from build123d import *


with BuildPart() as part:
    # Sketch1 → Revolve1 (revolve)
    with BuildSketch(Plane(origin=(0, 0, 0), x_dir=(0, 0, -1), z_dir=(1, 0, 0))):
        Polygon((-562.5, 225), (-562.5, -225), (0, -225), (0, -185), (0, 225), (0, 252.019037432), (-562.5, 252.019037432), align=None)
        Polygon((-30, -190), (-220, -190), (-220, -215), (-275, -215), (-275, -190), (-537.5, -190), (-537.5, 185), (-537.5, 225), (-30, 225), (-30, 185), align=None, mode=Mode.SUBTRACT)
    revolve(axis=Axis((0, 225, 0), (0, -1, 0)))


solid = part.part
The model under review builds one solid part; all positions refer to its coordinate system, in mm. A direction names the side the tool comes from. Round coordinates to 2 decimals unless told otherwise and drop trailing zeros. Loops run counter-clockwise (first coordinate to the right, second up) from the corner with the lowest first, then second, coordinate; pieces in that order, holes last. Notation, with made-up numbers: M 41,67 L 75,67 A10 cw 75,74 Z; hole C -22.75,59.5 d4. An arc over 180 degrees is marked long. Answer as CSV lines item,"result".
1. Insertion check: pin 1 Ø6 at (y, z) = (115.5, -178) entering from -X; pin 2 Ø10 at (x, y) = (170.5, 83.5) entering from +Z; pin 3 Ø12 at (y, z) = (115.5, -367) entering from -X. Each pin has a flat end and moves straight along its axis. Give the tip position at first contact, or say it passes through.
Outcome:
pin 1,"stops at x = -534.59"
pin 2,"stops at z = 537.6"
pin 3,"stops at x = -431.38"
2. We need section D-D (x = 354). Give the boundary of the cut face in (y, z).
Outcome:
outline,"M -225,-437.14 L 252.02,-437.14 L 252.02,437.14 L -225,437.14 Z; hole M -190,-404.46 L 225,-404.46 L 225,404.46 L -190,404.46 Z"
3. We need section B-B (x = 0). Give the boundary of the cut face in (y, z), plus the area to 3 significant figures.
Outcome:
outline,"M -225,-562.5 L 252.02,-562.5 L 252.02,562.5 L -225,562.5 Z; hole M -215,-275 L -190,-275 L -190,-537.5 L 225,-537.5 L 225,-30 L -190,-30 L -190,-220 L -215,-220 Z; hole M -215,220 L -190,220 L -190,30 L 225,30 L 225,537.5 L -190,537.5 L -190,275 L -215,275 Z"
area,"113,000 mm2"
4. To check wall thickness, follow L1, parallel to Z at x = 0, y = 81; L2, parallel to Z at x = 0, y = -209. State the ranges of each line that lie inside material, in increasing order. Write a range as [from, to].
Outcome:
L1,"z = [-562.5, -537.5], [-30, 30], [537.5, 562.5]"
L2,"z = [-562.5, -275], [-220, 220], [275, 562.5]"
5. For faces 1 (the face through (46, -190, 3)), 2 (the face through (-8, -225, -8)), list the 3-axis set-ups (+Z, -Z, +X, -X, +Y, -Y) from which the entire face can be reached by the end or side of a thin tool; tool diameter is ignored.
Outcome:
face 1,"none"
face 2,"+Z, -Z, +X, -X, -Y"
6. Draft analysis for pull direction Z (two halves, no side actions). For faces 3 (the face through (-8, 252.019, 8)), 4 (the face through (-82.6, -202.3, 262.3)), 5 (the face through (-168.96, 10.17, 536.525)), state which applies: pulls with the +Z half, pulls with the -Z half, needs draft (parallel to the pull), parting line crosses it, or undercut.
Outcome:
face 3,"needs draft"
face 4,"undercut"
face 5,"parting line crosses it"
7. We need section A-A (y = 75). Give the boundary of the cut face in (x, z).
Outcome:
outline,"C 0,0 d1125; C 0,0 d60; hole C 0,0 d1075"
8. We need section C-C (z = 0). Give the boundary of the cut face in (x, y), plus the area to 3 significant figures.
Outcome:
outline,"M -562.5,-225 L 562.5,-225 L 562.5,252.02 L -562.5,252.02 Z; hole M -537.5,-190 L -275,-190 L -275,-215 L -220,-215 L -220,-190 L -30,-190 L -30,225 L -537.5,225 Z; hole M 30,-190 L 220,-190 L 220,-215 L 275,-215 L 275,-190 L 537.5,-190 L 537.5,225 L 30,225 Z"
area,"113,000 mm2"
